Could you check a few things on this model? Use its own coordinates, in mm. Face numbers are marked on the shaded views. A direction names the side the tool comes from. Give positions to 0.01 mm unless a question says otherwise; leave off trailing zeros. Loops run counter-clockwise (first coordinate to the right, second up) from the corner with the lowest first, then second, coordinate; pieces in that order, holes last. Notation, with made-up numbers: M -35,46.5 L -16,46.5 A13 ccw -16,68.5 Z; hole C -29,22.25 d7. An arc over 180 degrees is marked long. Answer in a Markdown table with one row per item. Add a question column.
1. If we section it at A-A on z = 62.5: Count the separate pieces of the cut face and the enclosed holes in it, then the cut area to 3 significant figures.
2. Which directions (+Z, -Z, +X, -X, +Y, -Y) give clear straight access to the entire face, cutting with the end or side of a thin tool? Please do the marked faces 1 and 2.
3. If we section it at B-B on x = 140.5: List the corners of the cut face in (y, z) for me (3 decimals), then the cut area to 3 significant figures.
4. I'm going to push flat-ended pins straight in: pin 1 Ø1.5 at (x, z) = (105, 55) entering from +Y; pin 2 Ø5 at (x, y) = (336, 210.5) entering from +Z; pin 3 Ø8 at (x, z) = (9.5, 51) entering from -Y. Where does each tip first touch, or does it pass through?
5. If we section it at C-C on y = 170: List the corners of the cut face in (x, z) for me.
6. I need wall thicknesses on line 1 along X through (y, z) = (-43, 63); line 2 along Y through (x, z) = (-189.5, 20.5); line 3 along X through (y, z) = (134, 71.5). Which ranges of each line are inside material? Lowest first, please. Write a range as from..to.
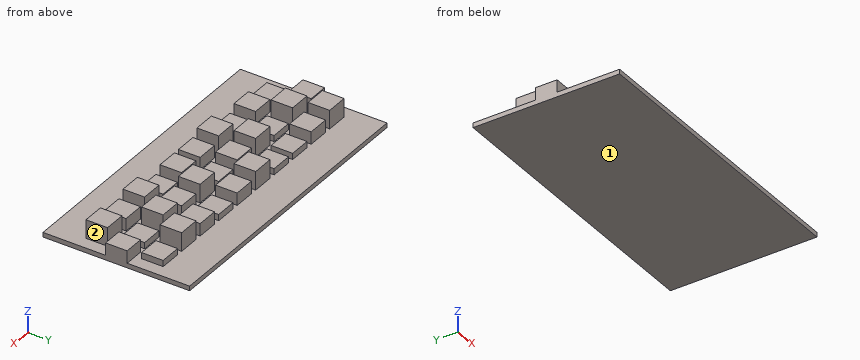
```python
from build123d import *

# Parameters (mm, degrees)
F0_W     = 88.9
F0_H     = 88.9
F0_W_2   = 82.55
F1_DEPTH = 19.05
F2_DEPTH = 25.4
F3_DEPTH = 76.2
F4_DEPTH = 50.8


with BuildPart() as f1:
    # F0 (on Top) → F1 (new body)
    with BuildSketch(Plane.XY):
        Polygon((609.6, 301.625), (-609.6, 301.625), (-609.6, 44.577), (-527.05, 44.577), (-527.05, -44.323), (-609.6, -44.323), (-609.6, -301.625), (609.6, -301.625), (609.6, -44.323), (527.05, -44.323), (527.05, 44.577), (609.6, 44.577), align=None)
        with Locations((-514.35, -114.173)):
            Rectangle(F0_W, F0_H, mode=Mode.SUBTRACT)
        with Locations((-400.05, -114.173)):
            Rectangle(F0_W, F0_H, mode=Mode.SUBTRACT)
        with Locations((-285.75, -114.173)):
            Rectangle(F0_W, F0_H, mode=Mode.SUBTRACT)
        with Locations((-171.45, -114.173)):
            Rectangle(F0_W, F0_H, mode=Mode.SUBTRACT)
        with Locations((-57.15, -114.173)):
            Rectangle(F0_W, F0_H, mode=Mode.SUBTRACT)
        with Locations((57.15, -114.173)):
            Rectangle(F0_W, F0_H, mode=Mode.SUBTRACT)
        with Locations((171.45, -114.173)):
            Rectangle(F0_W, F0_H, mode=Mode.SUBTRACT)
        with Locations((285.75, -114.173)):
            Rectangle(F0_W, F0_H, mode=Mode.SUBTRACT)
        with Locations((400.05, -114.173)):
            Rectangle(F0_W, F0_H, mode=Mode.SUBTRACT)
        with Locations((514.35, -114.173)):
            Rectangle(F0_W, F0_H, mode=Mode.SUBTRACT)
        with Locations((-457.2, 0.127)):
            Rectangle(F0_W, F0_H, mode=Mode.SUBTRACT)
        with Locations((-342.9, 0.127)):
            Rectangle(F0_W, F0_H, mode=Mode.SUBTRACT)
        with Locations((-514.35, 114.427)):
            Rectangle(F0_W, F0_H, mode=Mode.SUBTRACT)
        with Locations((-400.05, 114.427)):
            Rectangle(F0_W, F0_H, mode=Mode.SUBTRACT)
        with Locations((-228.6, 0.127)):
            Rectangle(F0_W, F0_H, mode=Mode.SUBTRACT)
        with Locations((-114.3, 0.127)):
            Rectangle(F0_W, F0_H, mode=Mode.SUBTRACT)
        with Locations((-285.75, 114.427)):
            Rectangle(F0_W, F0_H, mode=Mode.SUBTRACT)
        with Locations((-171.45, 114.427)):
            Rectangle(F0_W, F0_H, mode=Mode.SUBTRACT)
        with Locations((-57.15, 114.427)):
            Rectangle(F0_W, F0_H, mode=Mode.SUBTRACT)
        with Locations((0, 0.127)):
            Rectangle(F0_W, F0_H, mode=Mode.SUBTRACT)
        with Locations((114.3, 0.127)):
            Rectangle(F0_W, F0_H, mode=Mode.SUBTRACT)
        with Locations((228.6, 0.127)):
            Rectangle(F0_W, F0_H, mode=Mode.SUBTRACT)
        with Locations((57.15, 114.427)):
            Rectangle(F0_W, F0_H, mode=Mode.SUBTRACT)
        with Locations((171.45, 114.427)):
            Rectangle(F0_W, F0_H, mode=Mode.SUBTRACT)
        with Locations((285.75, 114.427)):
            Rectangle(F0_W, F0_H, mode=Mode.SUBTRACT)
        with Locations((342.9, 0.127)):
            Rectangle(F0_W, F0_H, mode=Mode.SUBTRACT)
        with Locations((457.2, 0.127)):
            Rectangle(F0_W, F0_H, mode=Mode.SUBTRACT)
        with Locations((400.05, 114.427)):
            Rectangle(F0_W, F0_H, mode=Mode.SUBTRACT)
        with Locations((514.35, 114.427)):
            Rectangle(F0_W, F0_H, mode=Mode.SUBTRACT)
        with Locations((-400.05, -114.173)):
            Rectangle(F0_W, F0_H)
        with Locations((-514.35, -114.173)):
            Rectangle(F0_W, F0_H)
        with Locations((-457.2, 0.127)):
            Rectangle(F0_W, F0_H)
        with Locations((-514.35, 114.427)):
            Rectangle(F0_W, F0_H)
        with Locations((-400.05, 114.427)):
            Rectangle(F0_W, F0_H)
        with Locations((-342.9, 0.127)):
            Rectangle(F0_W, F0_H)
        with Locations((-285.75, -114.173)):
            Rectangle(F0_W, F0_H)
        with Locations((-171.45, -114.173)):
            Rectangle(F0_W, F0_H)
        with Locations((-228.6, 0.127)):
            Rectangle(F0_W, F0_H)
        with Locations((-285.75, 114.427)):
            Rectangle(F0_W, F0_H)
        with Locations((-171.45, 114.427)):
            Rectangle(F0_W, F0_H)
        with Locations((-114.3, 0.127)):
            Rectangle(F0_W, F0_H)
        with Locations((-57.15, -114.173)):
            Rectangle(F0_W, F0_H)
        with Locations((57.15, -114.173)):
            Rectangle(F0_W, F0_H)
        with Locations((0, 0.127)):
            Rectangle(F0_W, F0_H)
        with Locations((-57.15, 114.427)):
            Rectangle(F0_W, F0_H)
        with Locations((57.15, 114.427)):
            Rectangle(F0_W, F0_H)
        with Locations((114.3, 0.127)):
            Rectangle(F0_W, F0_H)
        with Locations((171.45, -114.173)):
            Rectangle(F0_W, F0_H)
        with Locations((285.75, -114.173)):
            Rectangle(F0_W, F0_H)
        with Locations((228.6, 0.127)):
            Rectangle(F0_W, F0_H)
        with Locations((171.45, 114.427)):
            Rectangle(F0_W, F0_H)
        with Locations((342.9, 0.127)):
            Rectangle(F0_W, F0_H)
        with Locations((400.05, -114.173)):
            Rectangle(F0_W, F0_H)
        with Locations((285.75, 114.427)):
            Rectangle(F0_W, F0_H)
        with Locations((400.05, 114.427)):
            Rectangle(F0_W, F0_H)
        with Locations((457.2, 0.127)):
            Rectangle(F0_W, F0_H)
        with Locations((514.35, -114.173)):
            Rectangle(F0_W, F0_H)
        with Locations((514.35, 114.427)):
            Rectangle(F0_W, F0_H)
        with Locations((-568.325, 0.127)):
            Rectangle(F0_W_2, F0_H)
        with Locations((568.325, 0.127)):
            Rectangle(F0_W_2, F0_H)
    extrude(amount=-F1_DEPTH)

    # F0 (on Top) → F2 (join)
    with BuildSketch(Plane.XY):
        with Locations((514.35, 114.427)):
            Rectangle(F0_W, F0_H)
        with Locations((457.2, 0.127)):
            Rectangle(F0_W, F0_H)
        with Locations((171.45, -114.173)):
            Rectangle(F0_W, F0_H)
        with Locations((-514.35, -114.173)):
            Rectangle(F0_W, F0_H)
        with Locations((-342.9, 0.127)):
            Rectangle(F0_W, F0_H)
        with Locations((-285.75, -114.173)):
            Rectangle(F0_W, F0_H)
        with Locations((0, 0.127)):
            Rectangle(F0_W, F0_H)
        with Locations((171.45, 114.427)):
            Rectangle(F0_W, F0_H)
        with Locations((-285.75, 114.427)):
            Rectangle(F0_W, F0_H)
        with Locations((-171.45, 114.427)):
            Rectangle(F0_W, F0_H)
    extrude(amount=F2_DEPTH)

    # F0 (on Top) → F3 (join)
    with BuildSketch(Plane.XY):
        with Locations((514.35, -114.173)):
            Rectangle(F0_W, F0_H)
        with Locations((400.05, 114.427)):
            Rectangle(F0_W, F0_H)
        with Locations((342.9, 0.127)):
            Rectangle(F0_W, F0_H)
        with Locations((114.3, 0.127)):
            Rectangle(F0_W, F0_H)
        with Locations((-228.6, 0.127)):
            Rectangle(F0_W, F0_H)
        with Locations((-457.2, 0.127)):
            Rectangle(F0_W, F0_H)
        with Locations((285.75, -114.173)):
            Rectangle(F0_W, F0_H)
        with Locations((-171.45, -114.173)):
            Rectangle(F0_W, F0_H)
        with Locations((-514.35, 114.427)):
            Rectangle(F0_W, F0_H)
        with Locations((-57.15, 114.427)):
            Rectangle(F0_W, F0_H)
    extrude(amount=F3_DEPTH)

    # F0 (on Top) → F4 (join)
    with BuildSketch(Plane.XY):
        with Locations((-568.325, 0.127)):
            Rectangle(F0_W_2, F0_H)
        with Locations((-400.05, -114.173)):
            Rectangle(F0_W, F0_H)
        with Locations((-400.05, 114.427)):
            Rectangle(F0_W, F0_H)
        with Locations((57.15, 114.427)):
            Rectangle(F0_W, F0_H)
        with Locations((-114.3, 0.127)):
            Rectangle(F0_W, F0_H)
        with Locations((-57.15, -114.173)):
            Rectangle(F0_W, F0_H)
        with Locations((57.15, -114.173)):
            Rectangle(F0_W, F0_H)
        with Locations((228.6, 0.127)):
            Rectangle(F0_W, F0_H)
        with Locations((285.75, 114.427)):
            Rectangle(F0_W, F0_H)
        with Locations((400.05, -114.173)):
            Rectangle(F0_W, F0_H)
        with Locations((568.325, 0.127)):
            Rectangle(F0_W_2, F0_H)
    extrude(amount=F4_DEPTH)


solid = f1.part
```
Results:
| question | item | result |
|---|---|---|
| 1 | separate pieces | 10 |
| 1 | enclosed holes | 0 |
| 1 | area | 79,000 mm2 |
| 2 | face 1 | -Z, +X, -X, +Y, -Y |
| 2 | face 2 | +Z, +X, -Y |
| 3 | outline | M -301.625,-19.05 L 301.625,-19.05 L 301.625,0 L 158.877,0 L 158.877,25.4 L 69.977,25.4 L 69.977,0 L 44.577,0 L 44.577,76.2 L -44.323,76.2 L -44.323,0 L -69.723,0 L -69.723,25.4 L -158.623,25.4 L -158.623,0 L -301.625,0 Z |
| 3 | area | 22,800 mm2 |
| 4 | pin 1 | y = 44.58 |
| 4 | pin 2 | z = 0 |
| 4 | pin 3 | y = -158.62 |
| 5 | outline | M -609.6,-19.05 L 609.6,-19.05 L 609.6,0 L -609.6,0 Z |
| 6 | line 1 | -501.65..-412.75, -273.05..-184.15, 69.85..158.75, 298.45..387.35 |
| 6 | line 2 | -158.62..-69.72, -44.32..44.58, 69.98..158.88 |
| 6 | line 3 | -558.8..-469.9, -101.6..-12.7, 355.6..444.5 |
